Here's how the part is built. I have some questions about the finished solid (model axes, mm). Face numbers are marked on the shaded views. A direction names the side the tool comes from. Give positions to 0.01 mm unless a question says otherwise; leave off trailing zeros. Write each loop counter-clockwise with the first axis right and the second up, starting at its lowest first coordinate (ties: lowest second). Pieces come first, ordered by that corner, then holes. Notation, with made-up numbers: (17, -16) -> (42, -16) arc R23 cw to (42, -8) -> close; hole circle Ø7 at (65, 57.25). An arc over 180 degrees is marked (long way). Use one line per item in the form item = value.
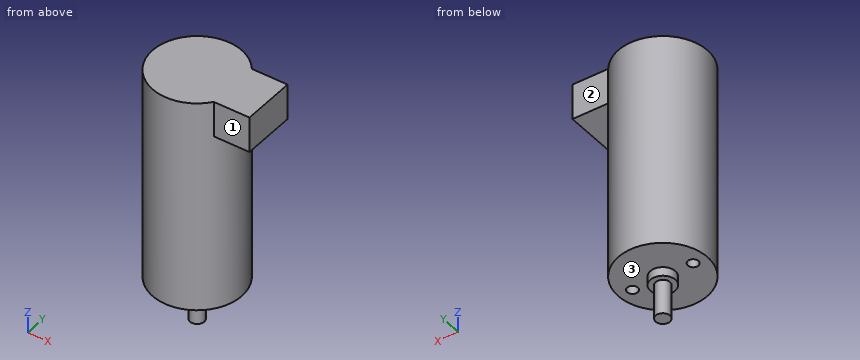
```python
from build123d import *

# Parameters (mm, degrees)
SKETCH1_R           = 12.5
BOSS_EXTRUDE1_DEPTH = 60
SKETCH2_R           = 1.5
CUT_EXTRUDE1_DEPTH  = 3.5
SKETCH2_3_R         = 3.5
SKETCH2_3_R_2       = 2
BOSS_EXTRUDE2_DEPTH = 2.5
SKETCH2_4_R         = 2
BOSS_EXTRUDE3_DEPTH = 12.2
SKETCH3_W           = 10
SKETCH3_H           = 15
BOSS_EXTRUDE4_DEPTH = 20


with BuildPart() as part:
    # Sketch1 → Boss-Extrude1 (new body)
    with BuildSketch(Plane.XY):
        Circle(SKETCH1_R)
    extrude(amount=BOSS_EXTRUDE1_DEPTH)

    # Sketch2 → Cut-Extrude1 (cut)
    with BuildSketch(Plane.XY):
        with Locations((8.5, 0)):
            Circle(SKETCH2_R)
        with Locations((-8.5, 0)):
            Circle(SKETCH2_R)
    extrude(amount=CUT_EXTRUDE1_DEPTH, mode=Mode.SUBTRACT)

    # Sketch2<3> → Boss-Extrude2 (add)
    with BuildSketch(Plane.XY):
        Circle(SKETCH2_3_R)
        Circle(SKETCH2_3_R_2, mode=Mode.SUBTRACT)
    extrude(amount=-BOSS_EXTRUDE2_DEPTH)

    # Sketch2<4> → Boss-Extrude3 (add)
    with BuildSketch(Plane.XY):
        Circle(SKETCH2_4_R)
    extrude(amount=-BOSS_EXTRUDE3_DEPTH)

    # Sketch3 → Boss-Extrude4 (add)
    with BuildSketch(Plane(origin=(0, 0, 0), x_dir=(0, 0, -1), z_dir=(1, 0, 0))):
        with Locations((-55, 0)):
            Rectangle(SKETCH3_W, SKETCH3_H)
    extrude(amount=BOSS_EXTRUDE4_DEPTH)


solid = part.part
```
Q1. I want a section at D-D, the plane x = 8.5. Write out the boundary of the cut face in (y, z), and give its area (3 significant figures).
Result set:
outline = (-9.17, 0) -> (-1.5, 0) -> (-1.5, 3.5) -> (1.5, 3.5) -> (1.5, 0) -> (9.17, 0) -> (9.17, 60) -> (-9.17, 60) -> close
area = 1,090 mm2
Q2. Which directions (+Z, -Z, +X, -X, +Y, -Y) give clear straight access to the entire face, cutting with the end or side of a thin tool? Please do the marked faces 1, 2 and 3.
Result set:
face_1 = +Z, -Z, +X, -Y
face_2 = +Z, -Z, +X, +Y
face_3 = -Z
Q3. Will these pins go through, and if not, where does the flat tip stop? pin 1 Ø1.5 at (x, y) = (-9, 0) entering from -Z; pin 2 Ø5 at (x, z) = (16, 52.5) entering from +Y; pin 3 Ø12 at (y, z) = (-8, -4.5) entering from +X.
Result set:
pin_1 = 3.5
pin_2 = 7.5
pin_3 = 11.83
Q4. I want a section at C-C, the plane y = 9.75. Write out the boundary of the cut face in (x, z), and give its area (3 significant figures).
Result set:
outline = (-7.82, 0) -> (7.82, 0) -> (7.82, 60) -> (-7.82, 60) -> close
area = 939 mm2
Q5. If I drill on line 1 along Z through (x, y) = (1.5, 2.25); line 2 along Z through (x, y) = (8.5, -5); line 3 along X through (y, z) = (-10, 47), over which ranges is the centre line in solid material (lowest first)? Write a range as from..to.
Result set:
line_1 = -2.5..60
line_2 = 0..60
line_3 = -7.5..7.5
Q6. I want a section at A-A, the plane x = 0. Write out the boundary of the cut face in (y, z), and give its area (3 significant figures).
Result set:
outline = (-12.5, 0) -> (-3.5, 0) -> (-3.5, -2.5) -> (-2, -2.5) -> (-2, -12.2) -> (2, -12.2) -> (2, -2.5) -> (3.5, -2.5) -> (3.5, 0) -> (12.5, 0) -> (12.5, 60) -> (-12.5, 60) -> close
area = 1,560 mm2
Q7. I want a section at B-B, the plane z = 46. Write out the boundary of the cut face in (x, y), and give its area (3 significant figures).
Result set:
outline = circle Ø25 at (0, 0)
area = 491 mm2
